from build123d import *

# Parameters (mm, degrees)
F1_R          = 11.5
F2_DEPTH      = 19.51505
F2_DEPTH_BACK = 10
F0_R          = 8.875
F3_DEPTH      = 25
F3_DEPTH_BACK = 25
F5_DEPTH      = 25
F5_DEPTH_BACK = 25
F6_W          = 31.0526300933
F6_H          = 13.8705706969
F6_H_2        = 13.1759493425
F7_DEPTH      = 25
F7_DEPTH_BACK = 25
F8_SIZE       = 0.5


with BuildPart() as f2:
    # F1 (on Top) → F2 (new body, two sides)
    with BuildSketch(Plane.XY) as f2_sk:
        Circle(F1_R)
    extrude(amount=F2_DEPTH)
    extrude(f2_sk.sketch, amount=-F2_DEPTH_BACK)

    # F0 (on Front) → F3 (cut, two sides)
    with BuildSketch(Plane.XZ) as f3_sk:
        Circle(F0_R)
    extrude(amount=-F3_DEPTH, mode=Mode.SUBTRACT)
    extrude(f3_sk.sketch, amount=F3_DEPTH_BACK, mode=Mode.SUBTRACT)

    # F4 (on Front) → F5 (cut, two sides)
    with BuildSketch(Plane.XZ) as f5_sk:
        Polygon((24.7668549418, 28.5545103252), (-16.3316316903, 28.5545103252), (24.7668549418, -1.7773286672), align=None)
    extrude(amount=-F5_DEPTH, mode=Mode.SUBTRACT)
    extrude(f5_sk.sketch, amount=F5_DEPTH_BACK, mode=Mode.SUBTRACT)

    # F6 (on Top) → F7 (cut, two sides)
    with BuildSketch(Plane.XY) as f7_sk:
        with Locations((1.910218969, 10.3145037405)):
            Rectangle(F6_W, F6_H)
        with Locations((1.910218969, -13.2087562792)):
            Rectangle(F6_W, F6_H_2)
    extrude(amount=-F7_DEPTH, mode=Mode.SUBTRACT)
    extrude(f7_sk.sketch, amount=F7_DEPTH_BACK, mode=Mode.SUBTRACT)

    # F8
    f8_edges = [f2.edges().sort_by_distance(p)[0] for p in [
        (-8.875, 3.379218, 0),
        (-8.875, -6.620782, 0),
    ]]
    chamfer(f8_edges, length=F8_SIZE)


solid = f2.part
The listing builds one solid part. Answer for the finished solid, in the listing's coordinates (mm). Coordinates: 2 decimals unless noted, no trailing zeros. Loops run counter-clockwise (first coordinate to the right, second up) from the corner with the lowest first, then second, coordinate; pieces in that order, holes last. Notation, with made-up numbers: (41, 5.5) -> (73, 5.5) arc R29 cw to (73, 34.5) -> close; hole circle Ø9 at (87.5, 45). An arc over 180 degrees is marked (long way). Write item = value, one per line. Start each with the question number.
1) A cutting plane is placed at D-D (z = 15.5). Give the vertices of the cut face in (x, y), then the cut area to 3 significant figures.
2) Straight lines are drawn through the part: line 1 (X direction, y = -3, z = -2.5); line 2 (Z direction, x = -3.75, y = -0.5); line 3 (X direction, y = -1.5, z = 0) (3 decimals). For each, find the intervals that lie inside material, in ascending order. Write a range as from..to.
3) Given pin 1 Ø1.5 at (x, z) = (5.5, -4.5) entering from +Y; pin 2 Ø2 at (y, z) = (-1.5, 15.5) entering from +X; pin 3 Ø1.5 at (y, z) = (-4, 11.5) entering from +X, each flat-ended and moving along its own axis, determine where each tip first touches the part or whether it passes through.
4) The mould has two halves that part along X. Classify faces 1 (the face through (-1.924, -1.684, -8.664)), 2 (the face through (11.346, -1.878, -0.082)), 3 (the face through (-8, -2, 19.515)): released by +X, released by -X, zero draft, split by the parting line, or undercut.
5) A cutting plane is placed at B-B (x = 0). Give the vertices of the cut face in (y, z) (3 decimals).
6) A cutting plane is placed at A-A (z = 0). Give the vertices of the cut face in (x, y) (3 decimals), then the cut area to 3 significant figures.
Responses:
q1.outline = (-10.99, 3.38) arc R11.5 ccw to (-9.4, -6.62) -> (1.36, -6.62) -> (1.36, 3.38) -> close
q1.area = 124 mm²
q2.line_1 = -11.1..-8.52, 8.52..11.1
q2.line_2 = -10..-8.04, 8.04..19.27
q2.line_3 = -11.402..-8.875, 8.875..11.402
q3.pin_1 = through
q3.pin_2 = 2.71
q3.pin_3 = 7.79
q4.face_1 = undercut
q4.face_2 = released by +X
q4.face_3 = zero draft
q5.outline = (-6.621, -10) -> (3.379, -10) -> (3.379, -9.375) -> (2.879, -8.875) -> (-6.121, -8.875) -> (-6.621, -9.375) -> close; (-6.621, 9.375) -> (-6.121, 8.875) -> (2.879, 8.875) -> (3.379, 9.375) -> (3.379, 16.501) -> (-6.621, 16.501) -> close
q6.outline = (-10.992, 3.379) arc R11.5 ccw to (-9.403, -6.621) -> (-9.375, -6.621) -> (-8.875, -6.121) -> (-8.875, 2.879) -> (-9.375, 3.379) -> close; (8.875, -6.121) -> (9.375, -6.621) -> (9.403, -6.621) arc R11.5 ccw to (10.992, 3.379) -> (9.375, 3.379) -> (8.875, 2.879) -> close
q6.area = 42.0 mm²
